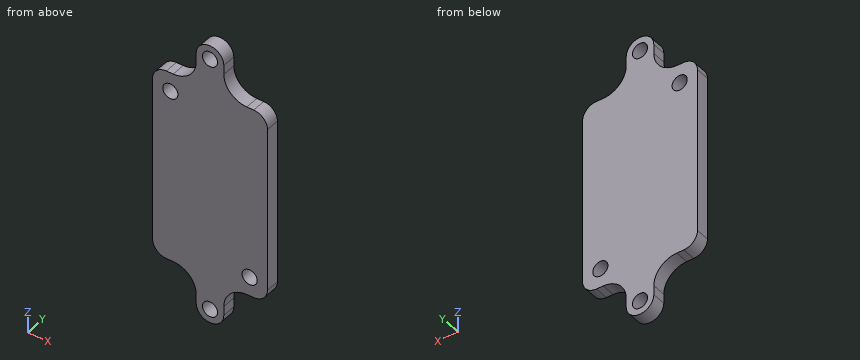
Autodesk Fusion 360 part; units mm, degrees
sketch "Sketch1" plane through (0, 0, 0) normal (0, 1, 0) x (1, 0, 0)
  line L0 (-12.5, 21) -> (12.5, 21)
  line L1 (12.5, 21) -> (12.5, -21)
  line L2 (12.5, -21) -> (-12.5, -21)
  line L3 (-12.5, -21) -> (-12.5, 21)
  line L4 (-12.5, 21) -> (12.5, -21) construction
  line L5 (12.5, 21) -> (-12.5, -21) construction
  line L6 (-8.625, 16.855) -> (8.625, 16.855) construction
  line L7 (8.625, 16.855) -> (8.625, -16.855) construction
  line L8 (8.625, -16.855) -> (-8.625, -16.855) construction
  line L9 (-8.625, -16.855) -> (-8.625, 16.855) construction
  line L10 (-8.625, 16.855) -> (8.625, -16.855) construction
  line L11 (8.625, 16.855) -> (-8.625, -16.855) construction
  circle A0 centre (8.625, 16.855) radius 1.65
  circle A1 centre (-8.625, -16.855) radius 1.65
  line L12 (0, 0) -> (0, 28) construction
  line L13 (0, 0) -> (0, -28) construction
  circle A2 centre (0, 28) radius 1.65
  line L14 (0, 28) -> (-1.65, 28) construction
  circle A3 centre (0, 28) radius 3
  line L15 (0, 28) -> (-3, 28)
  line L16 (-3, 28) -> (-3, 21)
  line L17 (3, 28) -> (3, 21)
  line L18 (-3, -28) -> (-3, -21)
  circle A4 centre (0, -28) radius 3
  line L19 (3, -28) -> (3, -21)
  circle A5 centre (0, -28) radius 1.65
  line L20 (0, 0) -> (12.5, 0) construction
  dimension "d1" = 25
  dimension "d2" = 42
  dimension "d3" = 17.25
  dimension "d4" = 33.71
  dimension "d9" = 3.3
  dimension "d10" = 3.3
  dimension "d13" = 28
  dimension "d14" = 28
  dimension "d15" = 3.3
  dimension "d17" = 6
extrude "Extrude2" add sketch "Sketch1" along normal blind 3
fillet "Fillet2" radius 3 4 edges at (12.5, 1.5, 21) (-12.5, 1.5, 21) (12.5, 1.5, -21) (-12.5, 1.5, -21)
fillet "Fillet3" radius 5 4 edges at (3, 1.5, 21) (-3, 1.5, 21) (-3, 1.5, -21) (3, 1.5, -21)
Geometry check sheet. Reference: the model listing, model coordinates, mm. Give positions to 0.01 mm unless a question says otherwise; leave off trailing zeros. Loops run counter-clockwise (first coordinate to the right, second up) from the corner with the lowest first, then second, coordinate; pieces in that order, holes last. Notation, with made-up numbers: M -19,51 L -15,51 A24 ccw -15,87 Z; hole C 74,-15 d6. An arc over 180 degrees is marked long. Write item = value, one per line.
(1) Gauge pin test, flat ends, axial feed: pin 1 Ø0.8 at (x, y) = (8.5, 2) entering from +Z; pin 2 Ø1.5 at (x, y) = (-2, 1.5) entering from +Z; pin 3 Ø0.6 at (y, z) = (1, 26.5) entering from +X; pin 4 Ø2 at (x, z) = (0, -28) entering from -Y. Record the tip position at first contact, or that the pin passes through.
Answer below:
pin_1 = 21
pin_2 = 30.73
pin_3 = 3
pin_4 = through
(2) Sectioned sample at A-A, the plane x = 0. Record the cut outline in (y, z), plus the area to 3 significant figures.
Answer below:
outline = M 0,-31 L 3,-31 L 3,-29.65 L 0,-29.65 Z; M 0,-26.35 L 3,-26.35 L 3,26.35 L 0,26.35 Z; M 0,29.65 L 3,29.65 L 3,31 L 0,31 Z
area = 166 mm2
(3) Material ranges on line 1 (X direction, y = 1.15, z = -28); line 2 (X direction, y = 1.2, z = 17); line 3 (Z direction, x = -8.25, y = 0.8), recorded low to high. Write a range as [from, to].
Answer below:
line_1 = [-3, -1.65], [1.65, 3]
line_2 = [-12.5, -10.27], [-6.98, 12.5]
line_3 = [-21, 15.25], [18.46, 21]
(4) Sectioned sample at B-B, the plane y = 1.2. Record the cut outline in (x, z) (3 decimals).
Answer below:
outline = M -12.5,-18 A3 ccw -9.5,-21 L -8,-21 A5 cw -3,-26 L -3,-28 A3 ccw 3,-28 L 3,-26 A5 cw 8,-21 L 9.5,-21 A3 ccw 12.5,-18 L 12.5,18 A3 ccw 9.5,21 L 8,21 A5 cw 3,26 L 3,28 A3 ccw -3,28 L -3,26 A5 cw -8,21 L -9.5,21 A3 ccw -12.5,18 Z; hole C -8.625,16.855 d3.3; hole C 0,-28 d3.3; hole C 0,28 d3.3; hole C 8.625,-16.855 d3.3
